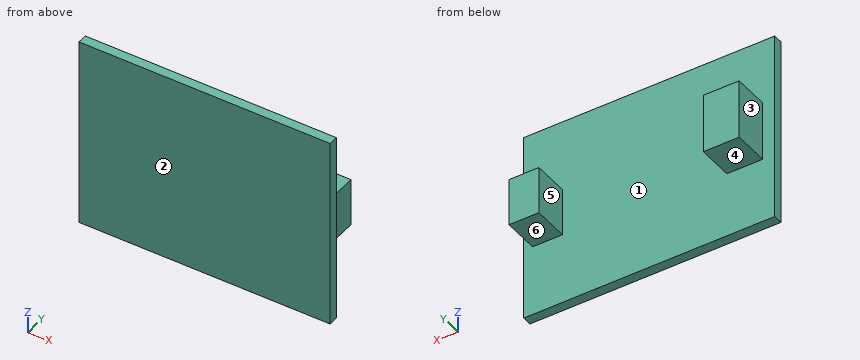
```python
from build123d import *

# Parameters (mm, degrees)
SKETCH1_W             = 42
SKETCH1_H             = 32
BOARD_DEPTH           = 1.6
PROBE_CONNECTOR_START = 1.6
SKETCH2_W             = 6
SKETCH2_H             = 10
PROBE_CONNECTOR_DEPTH = 6
SIGNAL_HEADER_START   = 1.6
SKETCH3_W             = 5
SKETCH3_H             = 8
SIGNAL_HEADER_DEPTH   = 6


with BuildPart() as part:
    # Sketch1 → Board (new body)
    with BuildSketch(Plane(origin=(0, 0, 0), x_dir=(1, 0, 0), z_dir=(0, 1, 0))):
        Rectangle(SKETCH1_W, SKETCH1_H)
    extrude(amount=BOARD_DEPTH)

    # Sketch2 → Probe_Connector (add)
    with BuildSketch(Plane(origin=(0, 0, 0), x_dir=(1, 0, 0), z_dir=(0, 1, 0)).offset(PROBE_CONNECTOR_START)):
        with Locations((-16, 0)):
            Rectangle(SKETCH2_W, SKETCH2_H)
    extrude(amount=PROBE_CONNECTOR_DEPTH)

    # Sketch3 → Signal_Header (add)
    with BuildSketch(Plane(origin=(0, 0, 0), x_dir=(1, 0, 0), z_dir=(0, 1, 0)).offset(SIGNAL_HEADER_START)):
        with Locations((17, 0)):
            Rectangle(SKETCH3_W, SKETCH3_H)
    extrude(amount=SIGNAL_HEADER_DEPTH)


solid = part.part
```
Here's how the part is built. I have some questions about the finished solid (model axes, mm). Face numbers are marked on the shaded views. A direction names the side the tool comes from. Coordinates: 2 decimals unless noted, no trailing zeros. Order: outer loops, then holes, each group sorted by start corner. A loop starts at its lowest first (then second) coordinate and runs counter-clockwise, first axis right, second up. Notation, with made-up numbers: (17.25, 9) -> (50.25, 9) arc R23 ccw to (50.25, 47) -> close; hole circle Ø6 at (15.5, 69). An arc over 180 degrees is marked (long way). Return JSON: item names as keys, results as strings.
1) If we section it at B-B on z = -2.5: List the corners of the cut face in (x, y) for me, plus the area to 3 significant figures.
Conclusion:
{"outline": "(-21, 0) -> (21, 0) -> (21, 1.6) -> (19.5, 1.6) -> (19.5, 7.6) -> (14.5, 7.6) -> (14.5, 1.6) -> (-13, 1.6) -> (-13, 7.6) -> (-19, 7.6) -> (-19, 1.6) -> (-21, 1.6) -> close", "area": "133 mm²"}
2) On a 3-axis mill with a long thin cutter (end or side, diameter ignored), from which of +Z, -Z, +X, -X, +Y, -Y can I reach the whole of each face in a straight line? I mean the marked faces 4, 5 and 6. Say none if no direction works.
Conclusion:
{"face 4": "-Z, +X, -X, +Y", "face 5": "+Z, -Z, +Y", "face 6": "-Z, +X, +Y"}
3) I'm going to push flat-ended pins straight in: P1, Ø3, axis at y = 6, z = 1.5, coming from the +X side; P2, Ø4, axis at x = 17.5, y = 4.5, coming from the -Z side; P3, Ø2.5, axis at x = 18, y = 4.5, coming from the +Z side. Where does each tip first touch, or does it pass through?
Conclusion:
{"P1": "stops at x = 19.5", "P2": "stops at z = -4", "P3": "stops at z = 4"}
4) If we section it at A-A on y = 6.5: List the corners of the cut face in (x, z) for me, plus the area to 3 significant figures.
Conclusion:
{"outline": "(-19, -5) -> (-13, -5) -> (-13, 5) -> (-19, 5) -> close; (14.5, -4) -> (19.5, -4) -> (19.5, 4) -> (14.5, 4) -> close", "area": "100 mm²"}
5) If we section it at C-C on x = -15: List the corners of the cut face in (y, z) for me.
Conclusion:
{"outline": "(0, -16) -> (1.6, -16) -> (1.6, -5) -> (7.6, -5) -> (7.6, 5) -> (1.6, 5) -> (1.6, 16) -> (0, 16) -> close"}
6) Thinking about a two-plate mould opening in X: for the marked faces 1, 2 and 3, which applies, +X half, -X half, draft (parallel to the pull), parting line (faces both ways), or undercut?
Conclusion:
{"face 1": "undercut", "face 2": "draft", "face 3": "-X half"}
7) If we section it at D-D on z = -12.5: List the corners of the cut face in (x, y) for me.
Conclusion:
{"outline": "(-21, 0) -> (21, 0) -> (21, 1.6) -> (-21, 1.6) -> close"}
8) If I drill on probe 1 along X at (y, z) = (7, 2.5); probe 2 along Y at (x, z) = (-8.5, -10.5); probe 3 along Z at (x, y) = (-14.5, 2.5), over which ranges is the centre line in solid material (lowest first)?
Conclusion:
{"probe 1": "x = -19 to -13, 14.5 to 19.5", "probe 2": "y = 0 to 1.6", "probe 3": "z = -5 to 5"}
